Check sheet for the modelled part. Datum: model origin and axes. Units: mm. Coordinates: 2 decimals unless noted, no trailing zeros. Order: outer loops, then holes, each group sorted by start corner. A loop starts at its lowest first (then second) coordinate and runs counter-clockwise, first axis right, second up.
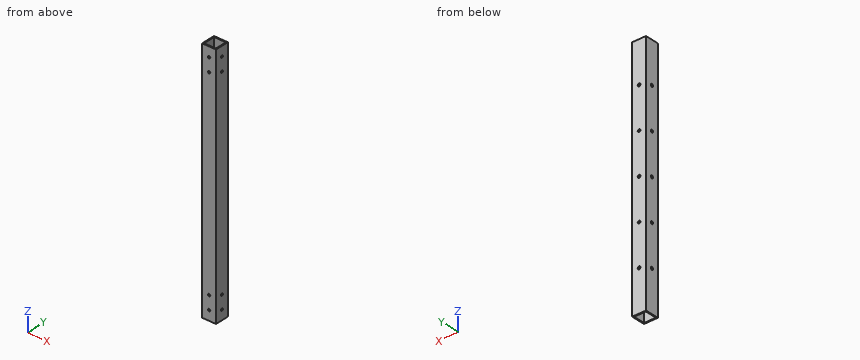
from build123d import *

# Parameters (mm, degrees)
SKETCH_1_W          = 25.4
SKETCH_1_H          = 25.4
EXTRUDE_1_DEPTH     = 450
SKETCH_1_3_W        = 21.4
SKETCH_1_3_H        = 21.4
CUT_EXTRUDE_1_DEPTH = 451.358279595
SKETCH_2_R          = 2.15
CUT_EXTRUDE_2_DEPTH = 3
SKETCH_3_R          = 2.15
CUT_EXTRUDE_3_DEPTH = 3
SKETCH_4_R          = 2.15
CUT_EXTRUDE_4_DEPTH = 3
SKETCH_5_R          = 2.15
CUT_EXTRUDE_5_DEPTH = 3
SKETCH_6_R          = 2.5
CUT_EXTRUDE_6_DEPTH = 10
SKETCH_8_R          = 2.5
CUT_EXTRUDE_7_DEPTH = 10


with BuildPart() as part:
    # Sketch 1 → Extrude 1 (new body)
    with BuildSketch(Plane.XY):
        Rectangle(SKETCH_1_W, SKETCH_1_H)
    extrude(amount=EXTRUDE_1_DEPTH)

    # Sketch 1_3 → Cut-Extrude 1 (cut, through all)
    with BuildSketch(Plane.XY):
        Rectangle(SKETCH_1_3_W, SKETCH_1_3_H)
    extrude(amount=CUT_EXTRUDE_1_DEPTH, mode=Mode.SUBTRACT)

    # Sketch 2 → Cut-Extrude 2 (cut)
    with BuildSketch(Plane.XZ.offset(12.7)):
        with Locations(Location((0, 17.7, 0), (0, 0, 270))):
            Circle(SKETCH_2_R)
        with Locations(Location((0, 42.2, 0), (0, 0, 270))):
            Circle(SKETCH_2_R)
    extrude(amount=-CUT_EXTRUDE_2_DEPTH, mode=Mode.SUBTRACT)

    # Sketch 3 → Cut-Extrude 3 (cut)
    with BuildSketch(Plane(origin=(12.7, 0, 0), x_dir=(0, 0, -1), z_dir=(1, 0, 0))):
        with Locations(Location((-42.2, 0, 0), (0, 0, 90))):
            Circle(SKETCH_3_R)
        with Locations(Location((-17.7, 0, 0), (0, 0, 90))):
            Circle(SKETCH_3_R)
    extrude(amount=-CUT_EXTRUDE_3_DEPTH, mode=Mode.SUBTRACT)

    # Sketch 4 → Cut-Extrude 4 (cut)
    with BuildSketch(Plane(origin=(12.7, 0, 0), x_dir=(0, 0, -1), z_dir=(1, 0, 0))):
        with Locations(Location((-407.8, 0, 0), (0, 0, 90))):
            Circle(SKETCH_4_R)
        with Locations(Location((-432.3, 0, 0), (0, 0, 90))):
            Circle(SKETCH_4_R)
    extrude(amount=-CUT_EXTRUDE_4_DEPTH, mode=Mode.SUBTRACT)

    # Sketch 5 → Cut-Extrude 5 (cut)
    with BuildSketch(Plane.XZ.offset(12.7)):
        with Locations(Location((0, 407.8, 0), (0, 0, 270))):
            Circle(SKETCH_5_R)
        with Locations(Location((0, 432.3, 0), (0, 0, 270))):
            Circle(SKETCH_5_R)
    extrude(amount=-CUT_EXTRUDE_5_DEPTH, mode=Mode.SUBTRACT)

    # Sketch 6 → Cut-Extrude 6 (cut)
    with BuildSketch(Plane(origin=(0, 12.7, 0), x_dir=(1, 0, 0), z_dir=(0, 1, 0))):
        with Locations(Location((0, -375, 0), (0, 0, 270))):
            Circle(SKETCH_6_R)
        with Locations(Location((0, -300, 0), (0, 0, 270))):
            Circle(SKETCH_6_R)
        with Locations(Location((0, -225, 0), (0, 0, 270))):
            Circle(SKETCH_6_R)
        with Locations(Location((0, -150, 0), (0, 0, 270))):
            Circle(SKETCH_6_R)
        with Locations(Location((0, -75, 0), (0, 0, 270))):
            Circle(SKETCH_6_R)
    extrude(amount=-CUT_EXTRUDE_6_DEPTH, mode=Mode.SUBTRACT)

    # Sketch 8 → Cut-Extrude 7 (cut)
    with BuildSketch(Plane.ZY.offset(12.7)):
        with Locations(Location((375, 0, 0), (0, 0, 270))):
            Circle(SKETCH_8_R)
        with Locations(Location((300, 0, 0), (0, 0, 270))):
            Circle(SKETCH_8_R)
        with Locations(Location((225, 0, 0), (0, 0, 270))):
            Circle(SKETCH_8_R)
        with Locations(Location((150, 0, 0), (0, 0, 270))):
            Circle(SKETCH_8_R)
        with Locations(Location((75, 0, 0), (0, 0, 270))):
            Circle(SKETCH_8_R)
    extrude(amount=-CUT_EXTRUDE_7_DEPTH, mode=Mode.SUBTRACT)


solid = part.part
(1) Go/stop test with a flat-tipped pin: P1, Ø5, axis at x = -3, y = 9.5, coming from the -Z side. Record where the tip stops, or that it passes through.
Filled in:
P1: stops at z = 0
(2) Cross-section at A-A (z = 108.5). Enter the section's corners in (x, y), and give its area (3 significant figures).
Filled in:
outline: (-12.7, -12.7) - (12.7, -12.7) - (12.7, 12.7) - (-12.7, 12.7) - close; hole (-10.7, -10.7) - (10.7, -10.7) - (10.7, 10.7) - (-10.7, 10.7) - close
area: 187 mm2
(3) Thickness scan on probe 1 along Z at (x, y) = (12.2, 0); probe 2 along X at (y, z) = (-6.5, 149). Record the ranges inside material, lowest first.
Filled in:
probe 1: z = 0 to 15.55, 19.85 to 40.05, 44.35 to 405.65, 409.95 to 430.15, 434.45 to 450
probe 2: x = -12.7 to -10.7, 10.7 to 12.7
